Autodesk Inventor part; units mm, degrees
ref_plane "YZ Plane" through (0, 0, 0) normal (1, 0, 0) x (0, 1, 0)
ref_plane "XZ Plane" through (0, 0, 0) normal (0, 1, 0) x (-1, 0, 0)
ref_plane "XY Plane" through (0, 0, 0) normal (0, 0, 1) x (1, 0, 0)
sketch "Sketch1" plane through (0, 0, 0) normal (0, 1, 0) x (-1, 0, 0)
  line L0 (0, 0) -> (56, 0)
  line L1 (56, 0) -> (56, -50)
  line L2 (56, -50) -> (0, -50)
  line L3 (0, -50) -> (0, 0)
  line L4 (56.2, 0) -> (-0.2, 0)
  line L5 (-0.2, 0) -> (-0.2, -50)
  line L6 (-0.2, -50) -> (56.2, -50)
  line L7 (56.2, -50) -> (56.2, 0)
  line L8 (58.7, 2.5) -> (-2.7, 2.5)
  line L9 (-2.7, 2.5) -> (-2.7, -52.5)
  line L10 (-2.7, -52.5) -> (58.7, -52.5)
  line L11 (58.7, -52.5) -> (58.7, 2.5)
  line L12 (56.2, -48.0985) -> (56.2, -52.5)
  line L13 (-0.2, -48.7936) -> (-0.2, -52.5)
  point P0 (-0.2, -50)
  dimension "d0" = 56
  dimension "d1" = 50
  dimension "d2" = 0.2
  dimension "d3" = 0.2
  dimension "d4" = 0
  dimension "d5" = 0
  dimension "d6" = 2.5
  dimension "d7" = 2.5
  dimension "d8" = 2.5
  dimension "d9" = 2.5
extrude "Extrusion1" add sketch "Sketch1" along normal blind 15.2 contours L4 L5 L13 L10 L9 L8 L11 L12 L7 L0
extrude "Extrusion2" add sketch "Sketch1" along normal blind 1
sketch "Sketch2" plane through (0.2, 15.2, 0) normal (0, 0, -1) x (-1, 0, 0)
  line L0 (0, -14.2) -> (0, 0)
  line L1 (0, -11.7) -> (56.4, -11.7)
  line L2 (56.4, -11.7) -> (56.4, -14.2)
  line L3 (56.4, -14.2) -> (0, -14.2)
  line L4 (0, -14.2) -> (0, -11.7)
  line L5 (56.4, -14.2) -> (56.4, 0)
  line L6 (0, -14.2) -> (56.4, -14.2)
  line L7 (1, -11.7) -> (55.4, -11.7)
  line L8 (55.4, -11.7) -> (55.4, -14.2)
  line L9 (55.4, -14.2) -> (1, -14.2)
  line L10 (1, -14.2) -> (1, -11.7)
  line L11 (0, -9) -> (56.4, -9)
  line L12 (56.4, -9) -> (56.4, -10)
  line L13 (56.4, -10) -> (0, -10)
  line L14 (0, -10) -> (0, -9)
  line L15 (56.4, -9) -> (55.4, -9)
  line L16 (55.4, -9) -> (55.4, -10)
  line L17 (55.4, -10) -> (56.4, -10)
  line L18 (56.4, -10) -> (56.4, -9)
  line L19 (0, -9) -> (1, -9)
  line L20 (1, -9) -> (1, -10)
  line L21 (1, -10) -> (0, -10)
  line L22 (0, -10) -> (0, -9)
  point P0 (0.2, -15.2)
  point P1 (0, -10)
  point P2 (1, -14.2)
  dimension "d14" = 0
  dimension "d16" = 2.5
  dimension "d17" = 1
  dimension "d18" = 1
  dimension "d19" = 0
  dimension "d20" = 0
  dimension "d21" = 1.7
  dimension "d22" = 1
extrude "Extrusion3" add sketch "Sketch2" along normal up to surface (52.5 mm away) contours L0 L1 L10 L3 | L0 L11 L20 L13 | L8 L1 L2 L3 | L16 L11 L5 L13
sketch "Sketch3" plane through (2.7, 0, -52.5) normal (0, 0, -1) x (-1, 0, 0)
  line L0 (2.5, 15.2) -> (58.9, 15.2)
  line L1 (23.5, 15.2) -> (43.9, 15.2)
  line L2 (43.9, 15.2) -> (43.9, 0)
  line L3 (43.9, 0) -> (23.5, 0)
  line L4 (23.5, 0) -> (23.5, 15.2)
  line L5 (58.9, 6.2) -> (58.9, 15.2)
  line L6 (2.5, 6.2) -> (2.5, 15.2)
  line L7 (0, 0) -> (61.4, 0)
  line L8 (23.5, 0) -> (43.9, 0)
  line L9 (43.9, 0) -> (43.9, 5)
  line L10 (43.9, 5) -> (23.5, 5)
  line L11 (23.5, 5) -> (23.5, 0)
  point P0 (2.7, 0)
  dimension "d25" = 15
  dimension "d26" = 21
  dimension "d27" = 0
  dimension "d30" = 5
extrude "Extrusion5" cut sketch "Sketch3" against normal blind 75.725 contours L10 L2 L3 L4
sketch "Sketch4" plane through (-58.7, 15.2, 2.5) normal (0, 0, 1) x (1, 0, 0)
  line L0 (11.5, -0.7) -> (20.5, -0.7)
  line L1 (20.5, -0.7) -> (20.5, -4.2)
  line L2 (20.5, -4.2) -> (11.5, -4.2)
  line L3 (11.5, -4.2) -> (11.5, -0.7)
  point P0 (58.7, -15.2)
  point P1 (3.5, -11.7)
  point P2 (2.5, -11.7)
  dimension "d33" = 7.5
  dimension "d34" = 11
  dimension "d35" = 18
  dimension "d36" = 9
extrude "Extrusion6" cut sketch "Sketch4" against normal up to surface (2.5 mm away)
sketch "Sketch5" plane through (0, 15.2, 0) normal (0, 1, 0) x (1, 0, 0)
  line L0 (2.7, -2.5) -> (2.7, 52.5)
  line L1 (2.7, -2.5) -> (2.7, 52.5)
  line L2 (2.7, 52.5) -> (0.2, 52.5)
  line L3 (2.7, 52.5) -> (0.2, 52.5)
  line L4 (0.2, 52.5) -> (0.2, 0)
  line L5 (0.2, 0) -> (-56.2, 0)
  line L6 (0.2, 0) -> (-56.2, 0)
  line L7 (-56.2, 52.5) -> (-58.7, 52.5)
  line L8 (-56.2, 0) -> (-56.2, 52.5)
  line L9 (-58.7, 52.5) -> (-58.7, -2.5)
  line L10 (-56.2, 52.5) -> (-58.7, 52.5)
  line L11 (-58.7, -2.5) -> (2.7, -2.5)
  line L12 (-58.7, 52.5) -> (-58.7, -2.5)
  line L13 (-58.7, -2.5) -> (2.7, -2.5)
  point P0 (0, 0)
extrude "Extrusion7" add sketch "Sketch5" along normal blind 3
sketch "Sketch6" plane through (0, 18.2, 0) normal (0, 1, 0) x (1, 0, 0)
  line L0 (2.7, -2.5) -> (2.7, 52.5)
  line L1 (-58.7, 52.5) -> (-58.7, -2.5)
  line L2 (2.7, -2.5) -> (-58.7, -2.5)
  line L3 (-58.7, -2.5) -> (-58.7, 52.5)
  line L4 (-58.7, 52.5) -> (2.7, 52.5)
  line L5 (2.7, 52.5) -> (2.7, -2.5)
  line L6 (-13.8, 42) -> (-1.8, 42)
  line L7 (-1.8, 42) -> (-1.8, 36)
  line L8 (-1.8, 36) -> (-13.8, 36)
  line L9 (-13.8, 36) -> (-13.8, 42)
  line L10 (0.2, 0) -> (-56.2, 0)
  line L11 (0.2, 52.5) -> (0.2, 0)
  line L12 (-10.8, 45) -> (-4.8, 45)
  line L13 (-13.8, 42) -> (-8.427, 47.373)
  line L14 (-13.8, 42) -> (-6.2015, 42) construction
  line L15 (-1.8, 42) -> (-7.8, 48)
  line L16 (-1.8, 42) -> (6.6853, 42) construction
  point P0 (0, 0)
  point P1 (-4.8, 45)
  point P2 (-58.7, -2.5)
  dimension "d41" = 36
  dimension "d42" = 42
  dimension "d43" = 2
  dimension "d44" = 14
  dimension "d45" = 3
  dimension "d46" = 3
  dimension "d47" = 45
  dimension "d48" = 135
  dimension "d49" = 3
extrude "Extrusion8" add sketch "Sketch6" along normal blind 1
sketch "Sketch7" plane through (2.7, 0, -52.5) normal (0, 0, -1) x (-1, 0, 0)
  line L0 (2.5, 3.5) -> (2.5, 5.2)
  line L1 (2.5, 3.5) -> (1.5, 3.5)
  line L2 (1.5, 3.5) -> (1.5, 5.2)
  line L3 (1.5, 5.2) -> (2.5, 5.2)
  line L4 (2.5, 5.2) -> (2.5, 3.5)
  line L5 (2.5, 6.2) -> (2.5, 18.2)
  line L6 (2.5, 18.2) -> (1.5, 18.2)
  line L7 (1.5, 18.2) -> (1.5, 6.2)
  line L8 (1.5, 6.2) -> (2.5, 6.2)
  line L9 (2.5, 6.2) -> (2.5, 18.2)
  line L10 (58.9, 3.5) -> (58.9, 5.2)
  line L11 (58.9, 3.5) -> (59.9, 3.5)
  line L12 (59.9, 3.5) -> (59.9, 5.2)
  line L13 (59.9, 5.2) -> (58.9, 5.2)
  line L14 (58.9, 5.2) -> (58.9, 3.5)
  line L15 (57.9, 6.2) -> (58.9, 6.2)
  line L16 (58.9, 6.2) -> (59.9, 6.2)
  line L17 (59.9, 6.2) -> (59.9, 18.2)
  line L18 (59.9, 18.2) -> (58.9, 18.2)
  line L19 (58.9, 18.2) -> (58.9, 6.2)
  point P0 (2.7, 0)
  dimension "d52" = 1
  dimension "d53" = 1
  dimension "d54" = 1
  dimension "d55" = 1
extrude "Extrusion9" cut sketch "Sketch7" against normal up to surface (52.5 mm away)
sketch "Sketch8" plane through (0, 19.2, 0) normal (0, 1, 0) x (1, 0, 0)
  line L0 (2.7, 52.5) -> (-20.8, 52.5)
  line L1 (-58.7, 52.5) -> (-58.7, -2.5)
  line L2 (2.7, 52.5) -> (-58.7, 52.5)
  line L3 (-58.7, 52.5) -> (-58.7, 49.5)
  line L4 (-58.7, 49.5) -> (2.7, 49.5)
  line L5 (2.7, 49.5) -> (2.7, 52.5)
  point P0 (0, 0)
  dimension "d58" = 3
extrude "Extrusion10" cut sketch "Sketch8" against normal up to surface (19.2 mm away)
sketch "Sketch9" plane through (0, 19.2, 0) normal (0, 1, 0) x (1, 0, 0)
  line L0 (2.7, -2.5) -> (2.7, 49.5)
  line L1 (-58.7, 49.5) -> (-58.7, -2.5)
  line L2 (2.7, 49.5) -> (-58.7, 49.5)
  line L3 (-58.7, 49.5) -> (-58.7, -2.5)
  line L4 (-58.7, -2.5) -> (2.7, -2.5)
  line L5 (2.7, -2.5) -> (2.7, 49.5)
  line L6 (-1.8, 42) -> (-1.8, 36)
  line L7 (-4.8, 45) -> (-1.8, 42)
  line L8 (-1.8, 42) -> (-4.8, 45)
  line L9 (-10.8, 45) -> (-4.8, 45)
  line L10 (-4.8, 45) -> (-10.8, 45)
  line L11 (-13.8, 42) -> (-10.8, 45)
  line L12 (-10.8, 45) -> (-13.8, 42)
  line L13 (-13.8, 36) -> (-13.8, 42)
  line L14 (-13.8, 42) -> (-13.8, 36)
  line L15 (-1.8, 36) -> (-13.8, 36)
  line L16 (-13.8, 36) -> (-1.8, 36)
  line L17 (-1.8, 36) -> (-1.8, 42)
  point P0 (0, 0)
extrude "Extrusion11" add sketch "Sketch9" along normal blind 1
sketch "Sketch10" plane through (1.2, 18.2, -49.5) normal (0, 0, -1) x (-1, 0, 0)
  line L0 (0, 0) -> (58.4, 0)
  line L1 (0, 0) -> (58.4, 0)
  line L2 (58.4, 0) -> (58.4, 1)
  line L3 (58.4, 1) -> (0, 1)
  line L4 (0, 1) -> (0, 0)
  point P0 (1.2, -18.2)
  dimension "d63" = 1
extrude "Extrusion12" cut sketch "Sketch10" against normal up to surface (49.5 mm away)
sketch "Sketch11" plane through (0, 20.2, 0) normal (0, 1, 0) x (1, 0, 0)
  line L0 (2.7, -2.5) -> (2.7, 49.5)
  line L1 (-58.7, 49.5) -> (-58.7, -2.5)
  line L2 (2.7, -2.5) -> (-58.7, -2.5)
  line L3 (-58.7, -2.5) -> (-58.7, -1)
  line L4 (-58.7, -1) -> (2.7, -1)
  line L5 (2.7, -1) -> (2.7, -2.5)
  point P0 (0, 0)
  dimension "d66" = 1.5
extrude "Extrusion13" cut sketch "Sketch11" against normal blind 24.925
sketch "Sketch12" plane through (-58.7, 20.2, 1) normal (0, 0, 1) x (1, 0, 0)
  line L0 (10.5, -3.7) -> (22.5, -3.7)
  line L1 (22.5, -3.7) -> (22.5, -11.2)
  line L2 (22.5, -11.2) -> (10.5, -11.2)
  line L3 (10.5, -11.2) -> (10.5, -3.7)
  line L4 (20.5, -5.7) -> (11.5, -5.7)
  line L5 (20.5, -9.2) -> (20.5, -5.7)
  line L6 (11.5, -9.2) -> (20.5, -9.2)
  line L7 (11.5, -5.7) -> (11.5, -9.2)
  point P0 (58.7, -20.2)
  dimension "d69" = 2
  dimension "d70" = 2
  dimension "d71" = 2
  dimension "d73" = 1
extrude "Extrusion14" cut sketch "Sketch12" against normal up to surface (1 mm away)
equation "\"d23\" = d16"
properties part number "case"
Read the model definition and answer for the solid it produces. Units are mm, in the model's axes. A direction names the side the tool comes from. Give positions to 0.01 mm unless a question says otherwise; leave off trailing zeros. Loops run counter-clockwise (first coordinate to the right, second up) from the corner with the lowest first, then second, coordinate; pieces in that order, holes last. Notation, with made-up numbers: (80.25, 52.25) - (115.25, 52.25) arc R6 ccw to (115.25, 62.25) - close; hole circle Ø10 at (-2.75, 1.5). An arc over 180 degrees is marked (long way). Answer as CSV lines item,"result". Start each with the question number.
1) Find section D-D (z = -11). Write down the section's boundary in (x, y), then the cut area to 3 significant figures.
2) Each of these flat-tipped pins is pushed along its axis until it touches: pin 1 Ø1.1 at (x, z) = (-40.5, 0.5) entering from -Y; pin 2 Ø5 at (x, z) = (-28, -31.5) entering from -Y; pin 3 Ø1.5 at (x, y) = (-22, 12.5) entering from -Z. Where does it stop, or does it pass through?
3) Straight lines are drawn through the part: L1, parallel to X at y = 11.75, z = -13.5; L2, parallel to Y at x = -18.5, z = -19; L3, parallel to Z at x = -31, y = 17.5. For each, find the intervals that lie inside material, in ascending order. Write a range as from..to.
4) Find section C-C (x = -10). Write down the section's boundary in (y, z).
5) Find section A-A (x = -37.5). Write down the section's boundary in (y, z), then the cut area to 3 significant figures.
6) Determine the mould class of faces 1 (the face through (0, 6.2, -25)), 2 (the face through (-50, 0, -24)), 3 (the face through (-3.3, 19.7, -43.5)) for opening direction Y: released by +Y, released by -Y, zero draft, split by the parting line, or undercut.
7) Which of the six approach directions +Z, -Z, +X, -X, +Y, -Y give full straight-line access (tool end or side, diameter ignored) to faces 4 (the face through (-9, 0, -24)), 5 (the face through (1.2, 4, -25))?
8) Find section B-B (y = 10.25). Write down the section's boundary in (x, z), then the cut area to 3 significant figures.
Findings below:
1,outline,"(-58.7, 0) - (-41.2, 0) - (-41.2, 1) - (-55.2, 1) - (-55.2, 3.5) - (-57.2, 3.5) - (-57.2, 5.2) - (-55.2, 5.2) - (-55.2, 6.2) - (-57.2, 6.2) - (-57.2, 19.2) - (1.2, 19.2) - (1.2, 6.2) - (-0.8, 6.2) - (-0.8, 5.2) - (1.2, 5.2) - (1.2, 3.5) - (-0.8, 3.5) - (-0.8, 1) - (-20.8, 1) - (-20.8, 0) - (2.7, 0) - (2.7, 20.2) - (-58.7, 20.2) - close"
1,area,"171 mm^2"
2,pin 1,"y = 5"
2,pin 2,"y = 19.2"
2,pin 3,"z = 0"
3,L1,"-58.7..-57.2, 1.2..2.7"
3,L2,"0..1, 19.2..20.2"
3,L3,"0..1"
4,outline,"(0, -49.5) - (1, -49.5) - (1, 0) - (19.2, 0) - (19.2, -36) - (20.2, -36) - (20.2, 1) - (0, 1) - close; (19.2, -49.5) - (20.2, -49.5) - (20.2, -45) - (19.2, -45) - close"
5,outline,"(5, 0) - (9, 0) - (9, 1) - (5, 1) - close; (16.5, 0) - (19.2, 0) - (19.2, -49.5) - (20.2, -49.5) - (20.2, 1) - (16.5, 1) - close"
5,area,"57.2 mm^2"
6,face 1,"undercut"
6,face 2,"released by -Y"
6,face 3,"zero draft"
7,face 4,"+Z, -Z, +X, -X, -Y"
7,face 5,"-Z"
8,outline,"(-58.7, -49.5) - (-57.2, -49.5) - (-57.2, 0) - (-48.2, 0) - (-48.2, 1) - (-58.7, 1) - close; (-36.2, 0) - (1.2, 0) - (1.2, -49.5) - (2.7, -49.5) - (2.7, 1) - (-36.2, 1) - close"
8,area,"198 mm^2"
